```python
from build123d import *

# Parameters (mm, degrees)
F3_R      = 14
F4_DEPTH  = 30
F6_R      = 4.5
F7_DEPTH  = 27
F5_R      = 7.75
F8_DEPTH  = 11
F10_DEPTH = 25


# Not quite as in the source:
# - a feature names something its author has since deleted; it is built from what else it names


with BuildPart() as f2:
    # F0 (on Front) → F2 (revolve)
    with BuildSketch(Plane.XZ):
        Polygon((32.2950072587, 0), (19.05, 38.1), (13.97, 38.1), (13.97, 0), align=None)
    revolve(axis=Axis((0, 0, 18.1650817394), (0, 0, 1)))

    # F3 (on Top) → F4 (join)
    with BuildSketch(Plane.XY):
        Circle(F3_R)
    extrude(amount=F4_DEPTH)

    # F6 (on face) → F7 (cut)
    with BuildSketch(Plane.XY.offset(30)):
        Circle(F6_R)
    extrude(amount=-F7_DEPTH, mode=Mode.SUBTRACT)

    # F5 (on face) → F8 (cut)
    with BuildSketch(Plane.XY.offset(30)):
        Circle(F5_R)
    extrude(amount=-F8_DEPTH, mode=Mode.SUBTRACT)

    # F9 (on face) → F10 (cut)
    with BuildSketch(Plane.XY.offset(30)):
        Polygon((-3.5, 0), (0, 0), (3.5, 0), (3.5, 10.5), (-3.5, 10.5), align=None)
    extrude(amount=-F10_DEPTH, mode=Mode.SUBTRACT)


solid = f2.part
```
Read the model definition and answer for the solid it produces. Units are mm, in the model's axes. A direction names the side the tool comes from. Coordinates: 2 decimals unless noted, no trailing zeros. Loops run counter-clockwise (first coordinate to the right, second up) from the corner with the lowest first, then second, coordinate; pieces in that order, holes last.
(1) Consider line 1 along Z through (x, y) = (-6, 9); line 2 along X through (y, z) = (-2.5, 22); line 3 along X through (y, z) = (5, 33.5). Determine where each line is inside the solid, lowest interval first.
Solution:
line 1: z = 0 to 30
line 2: x = -24.52 to -7.34, 7.34 to 24.52
line 3: x = -20.03 to -13.04, 13.04 to 20.03
(2) A tool of negligible diameter and unlimited length cuts with its end or side. For faces 4 (the face through (0, 0, 0)), 5 (the face through (-1.82, 13.85, 33.99)), from which of +Z, -Z, +X, -X, +Y, -Y can it reach the whole face along a straight path? Write none if from no direction.
Solution:
face 4: -Z, +X, -X, +Y, -Y
face 5: +Z
(3) The part is cut by section C-C (z = 15.5). Determine the outline of the cut face in (x, y).
Solution:
outline: circle Ø53.81 at (0, 0); hole (-3.5, 2.83) arc R4.5 ccw (long way) to (3.5, 2.83) - (3.5, 10.5) - (-3.5, 10.5) - close
(4) The part is cut by section D-D (z = 35). Determine the outline of the cut face in (x, y).
Solution:
outline: circle Ø40.26 at (0, 0); hole circle Ø27.94 at (0, 0)
(5) The mould has two halves that part along X. Classify faces 1 (the face through (-6, 13, 38.1)), 2 (the face through (2.08, -3.99, 11.11)), 3 (the face through (-5, -22, 28)): released by +X, released by -X, zero draft, split by the parting line, or undercut.
Solution:
face 1: zero draft
face 2: undercut
face 3: split by the parting line
(6) The part is cut by section A-A (x = 0). Determine the outline of the cut face in (y, z) (3 decimals).
Solution:
outline: (-32.295, 0) - (32.295, 0) - (19.05, 38.1) - (13.97, 38.1) - (13.97, 30) - (10.5, 30) - (10.5, 5) - (4.5, 5) - (4.5, 3) - (-4.5, 3) - (-4.5, 19) - (-7.75, 19) - (-7.75, 30) - (-13.97, 30) - (-13.97, 38.1) - (-19.05, 38.1) - close
(7) The part is cut by section B-B (y = 0). Determine the outline of the cut face in (x, z) (3 decimals), and give its area (3 significant figures).
Solution:
outline: (-32.295, 0) - (32.295, 0) - (19.05, 38.1) - (13.97, 38.1) - (13.97, 30) - (7.75, 30) - (7.75, 19) - (4.5, 19) - (4.5, 3) - (-4.5, 3) - (-4.5, 19) - (-7.75, 19) - (-7.75, 30) - (-13.97, 30) - (-13.97, 38.1) - (-19.05, 38.1) - close
area: 1,420 mm2
(8) Flat-ended cylindrical pins translate along their axes: pin 1 Ø2 at (x, z) = (9, 9.5) entering from -Y; pin 2 Ø8 at (x, z) = (15, 27.5) entering from -Y; pin 3 Ø8 at (x, y) = (0, 0) entering from -Z; pin 4 Ø4.5 at (x, y) = (-1.5, 2.5) entering from +Z. Find the tip coordinate at first contact, or state that the pin passes through.
Solution:
pin 1: stops at y = -28.04
pin 2: stops at y = -20.4
pin 3: stops at z = 0
pin 4: stops at z = 19
